Geometry: final body of the model. Coordinates: model frame, mm. Round coordinates to 2 decimals unless told otherwise and drop trailing zeros. Order: outer loops, then holes, each group sorted by start corner. A loop starts at its lowest first (then second) coordinate and runs counter-clockwise, first axis right, second up. Notation, with made-up numbers: M 88.5,53 L 110.5,53 A26 cw 110.5,86 Z; hole C 40.25,42.25 d11. An arc over 180 degrees is marked long. Put each result on its own line as item: value. Start each with the question number.
1) Section B-B, the plane y = 41. Return loops of the section in (x, z), then the cut area to 3 significant figures.
2) Section C-C, the plane x = 1. Count the separate pieces of the cut face and the enclosed holes in it, then the cut area to 3 significant figures.
3) Section D-D, the plane z = -49.5. Return loops of the section in (x, y).
4) Section A-A, the plane z = 0. Return loops of the section in (x, y).
5) First-contact query: P1, Ø8, axis at y = 26, z = -1.5, coming from the -X side; P2, Ø1.5, axis at x = 4.5, y = 5.5, coming from the -Z side; P3, Ø2, axis at x = 4, y = 22.5, coming from the -Z side; P4, Ø3, axis at x = 2.5, z = -45, coming from the -Y side. Flat tips, straight axial feed; report the tip coordinate or a pass-through.
6) Draft query along Y for faces 1 (the cylindrical face through (3.131, -37.523, -22.47)), 2 (the cylindrical face through (3.219, -27.954, -16.314)), 3 (the flat face through (3.13, 58.2, -55.18)). Return one class per face: pulls with the +Y half, pulls with the -Y half, needs draft (parallel to the pull), parting line crosses it, or undercut.
7) Material intervals for probe 1 along Z at (x, y) = (1, -28.5); probe 2 along Y at (x, z) = (3.75, -3.5); probe 3 along Y at (x, z) = (1, 2.5), sorted ascending. Write a range as [from, to].
Autodesk Inventor part; units mm, degrees
ref_plane "YZ Plane" through (0, 0, 0) normal (1, 0, 0) x (0, 1, 0)
ref_plane "XZ Plane" through (0, 0, 0) normal (0, 1, 0) x (-1, 0, 0)
ref_plane "XY Plane" through (0, 0, 0) normal (0, 0, 1) x (1, 0, 0)
sketch "Sketch1" plane through (0, 0, 0) normal (1, 0, 0) x (0, 1, 0)
  circle A0 centre (0, 0) radius 38.1 construction
  line L0 (27.94, -25.903) -> (27.94, -76.2) construction
  line L1 (27.94, -76.2) -> (-27.94, -76.2) construction
  line L2 (-27.94, -76.2) -> (-27.94, -25.903) construction
  line L3 (-30.1625, -17.4625) -> (30.1625, -17.4625) construction
  line L4 (30.1625, -17.4625) -> (30.1625, 17.4625) construction
  line L5 (30.1625, 17.4625) -> (-30.1625, 17.4625) construction
  line L6 (-30.1625, 17.4625) -> (-30.1625, -17.4625) construction
  line L7 (-30.1625, -17.4625) -> (30.1625, 17.4625) construction
  line L8 (30.1625, -17.4625) -> (-30.1625, 17.4625) construction
  circle A1 centre (30.1625, 17.4625) radius 2.5527 construction
  circle A2 centre (30.1625, -17.4625) radius 2.5527 construction
  circle A3 centre (-30.1625, -17.4625) radius 2.5527 construction
  circle A4 centre (-30.1625, 17.4625) radius 2.5527 construction
  point P0 (0, -76.2)
  dimension "d0" = 76.2
  dimension "d1" = 55.88
  dimension "d2" = 76.2
  dimension "d3" = 60.325
  dimension "d4" = 34.925
  dimension "d5" = 5.1054
  dimension "d6" = 5.1054
  dimension "d7" = 5.1054
  dimension "d8" = 5.1054
sketch "Sketch2" plane through (0, 0, 0) normal (1, 0, 0) x (0, 1, 0)
  line L0 (-30.1625, -17.4625) -> (30.1625, -17.4625) construction
  circle A0 centre (30.1625, -17.4625) radius 2.5527 construction
  circle A1 centre (-30.1625, -17.4625) radius 2.5527 construction
  line L1 (-30.1625, 17.4625) -> (-30.1625, -17.4625) construction
  circle A2 centre (-30.1625, 17.4625) radius 2.5527 construction
  line L2 (30.1625, -17.4625) -> (30.1625, 17.4625) construction
  line L3 (30.1625, -17.4625) -> (-30.1625, 17.4625) construction
  line L4 (30.1625, 17.4625) -> (-30.1625, 17.4625) construction
  line L5 (-30.1625, -17.4625) -> (30.1625, 17.4625) construction
  circle A3 centre (30.1625, 17.4625) radius 2.5527 construction
  circle A4 centre (0, 0) radius 38.1 construction
  line L6 (27.94, -25.903) -> (27.94, -76.2) construction
  line L7 (27.94, -76.2) -> (-27.94, -76.2) construction
  line L8 (-27.94, -76.2) -> (-27.94, -25.903) construction
  circle A5 centre (60.325, 0) radius 12.7 construction
  circle A6 centre (35.56, -51.3927) radius 14.2875
  circle A7 centre (35.56, -51.3927) radius 31.75 construction
  circle A8 centre (60.325, 0) radius 9.525
  circle A9 centre (60.325, 0) radius 22.225 construction
  circle A10 centre (30.1625, 17.4625) radius 8.9027 construction
  circle A11 centre (30.1625, -17.4625) radius 8.9027 construction
  circle A12 centre (-30.1625, -17.4625) radius 8.9027 construction
  circle A13 centre (-30.1625, 17.4625) radius 8.9027 construction
  line L9 (63.2628, 22.03) -> (31.3393, 26.2871)
  line L10 (-39.0652, 17.4625) -> (-39.0652, -17.4625)
  arc A14 (80.6974, -8.8835) -> (63.2628, 22.03) centre (60.325, 0) ccw
  arc A15 (31.3393, 26.2871) -> (31.8447, 26.2048) centre (30.1625, 17.4625) ccw
  arc A16 (-31.8447, 26.2048) -> (-39.0652, 17.4625) centre (-30.1625, 17.4625) ccw
  arc A17 (-39.0652, -17.4625) -> (-33.568, -25.6881) centre (-30.1625, -17.4625) ccw
  circle A18 centre (35.56, -51.3927) radius 25.4 construction
  circle A19 centre (17.331, -33.7048) radius 4.7625 construction
  circle A20 centre (32.8295, -73.6177) radius 4.8895 construction
  circle A21 centre (59.9927, -44.45) radius 4.7625 construction
  line L11 (80.6974, -8.8835) -> (64.3582, -46.3536)
  circle A22 centre (0, 0) radius 25.4
  circle A23 centre (0, 0) radius 31.75 construction
  line L12 (31.8447, 26.2048) -> (5.9993, 31.178)
  line L13 (-5.9993, 31.178) -> (-31.8447, 26.2048)
  arc A24 (5.9993, 31.178) -> (-5.9993, 31.178) centre (0, 0) ccw
  circle A25 centre (35.56, -51.3927) radius 29.9974 construction
  circle A26 centre (35.56, -51.3927) radius 20.6375 construction
  circle A27 centre (35.56, -51.3927) radius 7.62 construction
  line L14 (63.8721, -47.2125) -> (52.3707, -63.3638)
  arc A28 (63.8721, -47.2125) -> (64.3582, -46.3536) centre (59.9927, -44.45) ccw
  arc A29 (19.784, -64.6978) -> (-33.568, -25.6881) centre (-87.007, -154.7631) ccw
  arc A30 (19.784, -64.6978) -> (52.3707, -63.3638) centre (35.56, -51.3927) ccw
  point P0 (0, -76.2)
  point P1 (71.3235, -6.35)
  point P2 (71.3235, 6.35)
  point P3 (60.325, 12.7)
  point P4 (49.3265, 6.35)
  point P5 (49.3265, -6.35)
  point P6 (60.325, -12.7)
  point P7 (29.3562, -76.0235)
  point P8 (31.5932, 26.2532)
  dimension "d9" = 25.4
  dimension "d14" = 360
  dimension "d16" = 28.575
  dimension "d17" = 57.0484
  dimension "d19" = 63.5
  dimension "d20" = 19.05
  dimension "d23" = 6.35
  dimension "d43" = 360
  dimension "d45" = 9.525
  dimension "d46" = 9.779
  dimension "d47" = 9.525
  dimension "d56" = 50.8
  dimension "d57" = 6.35
  dimension "d58" = 44.45
  dimension "d60" = 76.2
  dimension "d65" = 59.9948
  dimension "d66" = 6.35
  dimension "d75" = 15.24
  dimension "d76" = 50.8
  dimension "d77" = 44.45
  dimension "d78" = 22.225
  dimension "d79" = 139.7
extrude "Extrusion1" add sketch "Sketch2" along normal blind 6.35 contours L12 A15 L9 | A14 L11 A28 L14 A30 A29 A17 L10 A16 L13 A24 L12 L9 | A22
hole "Hole3" at (0, 59.9927, -44.45) at (0, 30.1625, 17.4625) at (0, 30.1625, -17.4625) at (0, -30.1625, -17.4625) at (0, -30.1625, 17.4625) direction (1, 0, 0) diameter 4.9784 end through all
sketch "Sketch6" plane through (6.35, 0, 0) normal (1, 0, 0) x (0, 0, -1)
  circle A0 centre (0, 0) radius 7.9375
  dimension "d80" = 15.875
extrude "Extrusion5" cut sketch "Sketch6" against normal blind 6.35
sketch "Sketch7" plane through (6.35, 0, 0) normal (1, 0, 0) x (0, 0, -1)
  line L0 (-22.8953, 0) -> (22.8953, 0) construction
  point P0 (0, 0)
  point P1 (0, 0)
  dimension "d83" = 45.7905
hole "Hole4" at (6.35, 0, 22.8953) at (6.35, 0, -22.8953) direction (-1, 0, 0) diameter 4.3434 end through all
properties part number "AR-007" material "Aluminum 6061"
Result sheet:
1. outline: M 0,-71.3 L 6.35,-71.3 L 6.35,-64.6 L 0,-64.6 Z; M 0,-38.18 L 6.35,-38.18 L 6.35,25 L 0,25 Z
1. area: 444 mm2
2. separate pieces: 1
2. enclosed holes: 10
2. area: 7,620 mm2
3. outline: M 0,4.84 L 6.35,4.84 L 6.35,21.4 L 0,21.4 Z; M 0,49.72 L 6.35,49.72 L 6.35,62.24 L 0,62.24 Z
4. outline: M 0,-39.07 L 6.35,-39.07 L 6.35,-7.94 L 0,-7.94 Z; M 0,7.94 L 6.35,7.94 L 6.35,50.8 L 0,50.8 Z; M 0,69.85 L 6.35,69.85 L 6.35,82.55 L 0,82.55 Z
5. P1: stops at x = 0
5. P2: stops at z = -50.75
5. P3: stops at z = -68.14
5. P4: stops at y = -2.53
6. face 1: pulls with the -Y half
6. face 2: undercut
6. face 3: pulls with the +Y half
7. probe 1: z = [-27.9, -19.32], [-15.61, 15.61], [19.32, 26.85]
7. probe 2: y = [-39.07, -7.12], [7.12, 51.47], [69.18, 82.27]
7. probe 3: y = [-39.07, -7.53], [7.53, 51.13], [69.52, 82.41]
